Verification items for the finished model (mm, model axes). Round coordinates to 2 decimals unless told otherwise and drop trailing zeros. Loops run counter-clockwise (first coordinate to the right, second up) from the corner with the lowest first, then second, coordinate; pieces in that order, holes last. Notation, with made-up numbers: M 36.5,64 L 95.5,64 A18 ccw 95.5,95 Z; hole C -37.5,33 d1. An arc over 180 degrees is marked long. Answer as CSV lines item,"result".
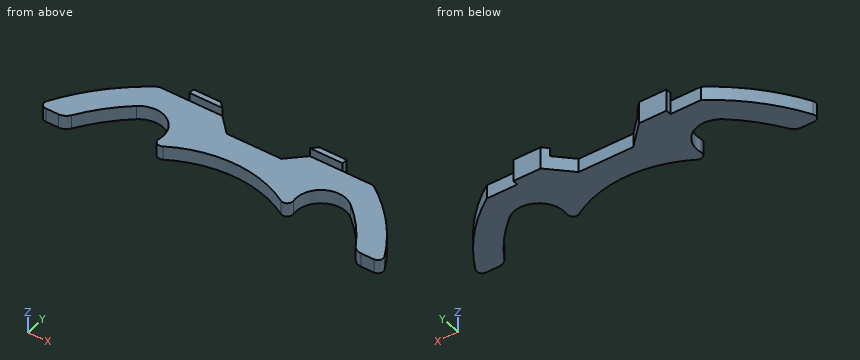
```python
from build123d import *

# Parameters (mm, degrees)
EXTRUSION1_DEPTH = 1.25
EXTRUSION2_DEPTH = 4


with BuildPart() as part:
    # Esquisse1 → Extrusion1 (new, symmetric)
    with BuildSketch(Plane.XY):
        with BuildLine():
            Line((-19.595917942, 29), (-8, 29))
            Line((-8, 29), (-5, 26))
            Line((-5, 26), (5, 26))
            Line((5, 26), (8, 29))
            Line((8, 29), (19.595917942, 29))
            ThreePointArc((19.595917942, 29), (26.005009087, 23.425189484), (30.882352941, 16.470588235))
            ThreePointArc((30.882352941, 16.470588235), (30.857492926, 15.485504245), (30, 15))
            Line((30, 15), (27.699277969, 15))
            ThreePointArc((27.699277969, 15), (26.722627492, 15.254676578), (25.994707017, 15.953846154))
            ThreePointArc((25.994707017, 15.953846154), (23.098976948, 19.917009413), (19.605022095, 23.364355515))
            ThreePointArc((19.605022095, 23.364355515), (14.428703263, 23.794573944), (12.29508997, 19.058852366))
            ThreePointArc((12.29508997, 19.058852366), (11.88737091, 18.049208847), (10.799200573, 18.01047659))
            ThreePointArc((10.799200573, 18.01047659), (0, 21), (-10.799200573, 18.01047659))
            ThreePointArc((-10.799200573, 18.01047659), (-11.88737091, 18.049208847), (-12.29508997, 19.058852366))
            ThreePointArc((-12.29508997, 19.058852366), (-14.428703263, 23.794573944), (-19.605022095, 23.364355515))
            ThreePointArc((-19.605022095, 23.364355515), (-23.098976948, 19.917009413), (-25.994707017, 15.953846154))
            ThreePointArc((-25.994707017, 15.953846154), (-26.722627492, 15.254676578), (-27.699277969, 15))
            Line((-27.699277969, 15), (-30, 15))
            ThreePointArc((-30, 15), (-30.857492926, 15.485504245), (-30.882352941, 16.470588235))
            ThreePointArc((-30.882352941, 16.470588235), (-26.005009087, 23.425189484), (-19.595917942, 29))
        make_face()
    extrude(amount=EXTRUSION1_DEPTH, both=True)

    # Esquisse2 → Extrusion2 (add)
    with BuildSketch(Plane(origin=(0, 0, -1.25), x_dir=(-1, 0, 0), z_dir=(0, 0, -1))):
        Polygon((-8, 29), (-14, 29), (-14, 30), (-9, 30), align=None)
        Polygon((8, 29), (9, 30), (14, 30), (14, 29), align=None)
    extrude(amount=-EXTRUSION2_DEPTH)


solid = part.part
```
1) Material ranges on probe 1 along X at (y, z) = (24, 0.2); probe 2 along X at (y, z) = (19.25, 0.75); probe 3 along Z at (x, y) = (-26, 21.75), recorded low to high.
Here are the results:
probe 1,"x = -25.48 to -18.6, -14.82 to 14.82, 18.6 to 25.48"
probe 2,"x = -29.23 to -23.66, -12.26 to -8.39, 8.39 to 12.26, 23.66 to 29.23"
probe 3,"z = -1.25 to 1.25"
2) Go/stop test with flat-tipped pins: pin 1 (0.8 mm diameter, centred on y = 29.5, z = 1.5, fed in from -X); pin 2 (8 mm diameter, centred on x = -24, y = 22.5, fed in from +Z); pin 3 (1.2 mm diameter, centred on x = -15.5, z = -0.5, fed in from +Y). Record where each tip stops, or that it passes through.
Here are the results:
pin 1,"stops at x = -14"
pin 2,"stops at z = 1.25"
pin 3,"stops at y = 29"
3) Section check B-B (y = 28). Record the cut outline in (x, z), plus the area to 3 significant figures.
Here are the results:
outline,"M -21,-1.25 L -7,-1.25 L -7,1.25 L -21,1.25 Z; M 7,-1.25 L 21,-1.25 L 21,1.25 L 7,1.25 Z"
area,"70.0 mm^2"
4) Section check A-A (z = 1.9). Record the cut outline in (x, y).
Here are the results:
outline,"M -14,29 L -8,29 L -9,30 L -14,30 Z; M 8,29 L 14,29 L 14,30 L 9,30 Z"
5) Section check C-C (y = 22.5). Record the cut outline in (x, z).
Here are the results:
outline,"M -26.81,-1.25 L -20.59,-1.25 L -20.59,1.25 L -26.81,1.25 Z; M -13.03,-1.25 L 13.03,-1.25 L 13.03,1.25 L -13.03,1.25 Z; M 20.59,-1.25 L 26.81,-1.25 L 26.81,1.25 L 20.59,1.25 Z"
6) Section check D-D (x = 2). Record the cut outline in (y, z), plus the area to 3 significant figures.
Here are the results:
outline,"M 20.9,-1.25 L 26,-1.25 L 26,1.25 L 20.9,1.25 Z"
area,"12.7 mm^2"
